from build123d import *

# Parameters (mm, degrees)
SKETCH1_W                     = 32.5
SKETCH1_H                     = 12.4
BOSS_EXTRUDE1_DEPTH           = 5
SKETCH3_W                     = 4.5
SKETCH3_H                     = 12.4
BOSS_EXTRUDE2_DEPTH           = 15.8
SKETCH4_R                     = 1
CUT_EXTRUDE1_DEPTH            = 5
SKETCH5_R                     = 1
BOSS_EXTRUDE3_DEPTH           = 2
BOSS_EXTRUDE3_DRAFT           = 5
BOSS_EXTRUDE3_PROFILE_2_DEPTH = 2
BOSS_EXTRUDE3_PROFILE_2_DRAFT = 5
BOSS_EXTRUDE3_PROFILE_3_DEPTH = 2
BOSS_EXTRUDE3_PROFILE_3_DRAFT = 5
SKETCH6_R                     = 4
BOSS_EXTRUDE4_DEPTH           = 1
SKETCH7_R                     = 1.5
BOSS_EXTRUDE5_DEPTH           = 5
FILLET1_R                     = 1
FILLET2_R                     = 1
FILLET3_R                     = 0.5
SKETCH10_W                    = 1.5
SKETCH10_H                    = 3
CUT_EXTRUDE4_DEPTH            = 34.527041325


with BuildPart() as part:
    # Sketch1 → Boss-Extrude1 (new body)
    with BuildSketch(Plane(origin=(0, 0, 0), x_dir=(1, 0, 0), z_dir=(0, 1, 0))):
        Rectangle(SKETCH1_W, SKETCH1_H)
    extrude(amount=BOSS_EXTRUDE1_DEPTH)

    # Sketch3 → Boss-Extrude2 (add)
    with BuildSketch(Plane(origin=(0, 5, 0), x_dir=(1, 0, 0), z_dir=(0, 1, 0))):
        with Locations((-14, 0)):
            Rectangle(SKETCH3_W, SKETCH3_H)
        with Locations((14, 0)):
            Rectangle(SKETCH3_W, SKETCH3_H)
    extrude(amount=BOSS_EXTRUDE2_DEPTH)

    # Sketch4 → Cut-Extrude1 (cut)
    with BuildSketch(Plane(origin=(0, 20.8, 0), x_dir=(1, 0, 0), z_dir=(0, 1, 0))):
        with Locations(Location((14.1, -0.06, 0), (0, 0, 270))):
            Circle(SKETCH4_R)
        with Locations(Location((-14.1, -0.06, 0), (0, 0, 270))):
            Circle(SKETCH4_R)
    extrude(amount=-CUT_EXTRUDE1_DEPTH, mode=Mode.SUBTRACT)


with BuildPart() as boss_extrude3_tool:
    # Sketch5 → Boss-Extrude3 (with draft: the straight prism first)
    with BuildSketch(Plane(origin=(16.25, 0, 0), x_dir=(0, 0, -1), z_dir=(1, 0, 0))):
        with Locations((0, 17.8)):
            Circle(SKETCH5_R)
    extrude(amount=BOSS_EXTRUDE3_DEPTH)
    # Boss-Extrude3: the draft: its side faces are tilted about the plane it starts from
    boss_extrude3_sides = [boss_extrude3_tool.faces().sort_by_distance(p)[0] for p in [
        (17.25, 17.8, 1),
    ]]
    draft(boss_extrude3_sides, Plane(origin=(16.25, 0, 0), x_dir=(0, 0, -1), z_dir=(1, 0, 0)), BOSS_EXTRUDE3_DRAFT)


with BuildPart() as part_1:
    add(part.part)

    # Boss-Extrude3: add boss_extrude3_tool
    add(boss_extrude3_tool.part)


with BuildPart() as boss_extrude3_profile_2_tool:
    # Sketch5 → Boss-Extrude3 profile 2 (with draft: the straight prism first)
    with BuildSketch(Plane(origin=(16.25, 0, 0), x_dir=(0, 0, -1), z_dir=(1, 0, 0))):
        with Locations((3.2, 12.8)):
            Circle(SKETCH5_R)
    extrude(amount=BOSS_EXTRUDE3_PROFILE_2_DEPTH)
    # Boss-Extrude3 profile 2: the draft: its side faces are tilted about the plane it starts from
    boss_extrude3_profile_2_sides = [boss_extrude3_profile_2_tool.faces().sort_by_distance(p)[0] for p in [
        (17.25, 12.8, -2.2),
    ]]
    draft(boss_extrude3_profile_2_sides, Plane(origin=(16.25, 0, 0), x_dir=(0, 0, -1), z_dir=(1, 0, 0)), BOSS_EXTRUDE3_PROFILE_2_DRAFT)


with BuildPart() as part_2:
    add(part_1.part)

    # Boss-Extrude3 profile 2: add boss_extrude3_profile_2_tool
    add(boss_extrude3_profile_2_tool.part)


with BuildPart() as boss_extrude3_profile_3_tool:
    # Sketch5 → Boss-Extrude3 profile 3 (with draft: the straight prism first)
    with BuildSketch(Plane(origin=(16.25, 0, 0), x_dir=(0, 0, -1), z_dir=(1, 0, 0))):
        with Locations((-3.2, 12.8)):
            Circle(SKETCH5_R)
    extrude(amount=BOSS_EXTRUDE3_PROFILE_3_DEPTH)
    # Boss-Extrude3 profile 3: the draft: its side faces are tilted about the plane it starts from
    boss_extrude3_profile_3_sides = [boss_extrude3_profile_3_tool.faces().sort_by_distance(p)[0] for p in [
        (17.25, 12.8, 4.2),
    ]]
    draft(boss_extrude3_profile_3_sides, Plane(origin=(16.25, 0, 0), x_dir=(0, 0, -1), z_dir=(1, 0, 0)), BOSS_EXTRUDE3_PROFILE_3_DRAFT)


with BuildPart() as part_3:
    add(part_2.part)

    # Boss-Extrude3 profile 3: add boss_extrude3_profile_3_tool
    add(boss_extrude3_profile_3_tool.part)

    # Sketch6 → Boss-Extrude4 (add)
    with BuildSketch(Plane.ZY.offset(16.25)):
        with Locations(Location((0, 17.8, 0), (0, 0, 131.409622109))):
            Circle(SKETCH6_R)
    extrude(amount=BOSS_EXTRUDE4_DEPTH)

    # Sketch7 → Boss-Extrude5 (add)
    with BuildSketch(Plane.ZY.offset(17.25)):
        with Locations((0, 17.8)):
            Circle(SKETCH7_R)
    extrude(amount=BOSS_EXTRUDE5_DEPTH)

    # Fillet1
    fillet1_edges = [part_3.edges().sort_by_distance(p)[0] for p in [
        (-22.25, 17.8, -1.5),
    ]]
    fillet(fillet1_edges, radius=FILLET1_R)

    # Fillet2
    fillet2_edges = [part_3.edges().sort_by_distance(p)[0] for p in [
        (-17.25, 14.8, 2.645751311),
    ]]
    fillet(fillet2_edges, radius=FILLET2_R - 0.0001)  # a hair under: the kernel refuses the full size

    # Fillet3
    fillet3_edges = [part_3.edges().sort_by_distance(p)[0] for p in [
        (18.25, 17.8, 0.825022673),
        (18.25, 12.8, -2.374977327),
        (18.25, 12.8, 4.025022673),
    ]]
    fillet(fillet3_edges, radius=FILLET3_R)

    # Sketch10 → Cut-Extrude4 (cut, through all)
    with BuildSketch(Plane(origin=(0, 0, -6.2), x_dir=(-1, 0, 0), z_dir=(0, 0, -1))):
        with Locations((-12.5, 9)):
            Rectangle(SKETCH10_W, SKETCH10_H)
    extrude(amount=-CUT_EXTRUDE4_DEPTH, mode=Mode.SUBTRACT)


solid = part_3.part
Read the model definition and answer for the solid it produces. Units are mm, in the model's axes. A direction names the side the tool comes from. Round coordinates to 2 decimals unless told otherwise and drop trailing zeros. Write each loop counter-clockwise with the first axis right and the second up, starting at its lowest first coordinate (ties: lowest second). Pieces come first, ordered by that corner, then holes.
1. The part is cut by section A-A, the plane z = 5.25. Determine the outline of the cut face in (x, y), then the cut area to 3 significant figures.
2. Determine the mould class of faces 5 (the face through (13.25, 9, 0)), 6 (the face through (-19.222, 16.336, -0.325)), 7 (the face through (14, 15.8, 0)) for opening direction Z: pulls with the +Z half, pulls with the -Z half, needs draft (parallel to the pull), parting line crosses it, or undercut.
3. Straight lines are drawn through the part: L1, parallel to X at y = 9, z = 0; L2, parallel to Y at x = 12, z = -1.5; L3, parallel to X at y = 12.5, z = 1.25. For each, find the intervals that lie inside material, in ascending order.
4. Given pin 1 Ø1.6 at (x, z) = (14.5, -0.5) entering from +Y; pin 2 Ø6 at (y, z) = (7.5, 0) entering from -X; pin 3 Ø6 at (x, z) = (0.5, 2) entering from +Y, each flat-ended and moving along its own axis, determine where each tip first touches the part or whether it passes through.
5. The part is cut by section C-C, the plane y = 1.5. Determine the outline of the cut face in (x, z).
6. Which of the six approach directions +Z, -Z, +X, -X, +Y, -Y give full straight-line access (tool end or side, diameter ignored) to faces 1 (the face through (13, 7.5, 0)), 2 (the face through (11.75, 16, 0)), 3 (the face through (-13.11, 18.34, -0.07)), 4 (the face through (-16.25, 21, 0))?
7. The part is cut by section B-B, the plane x = 14.1. Determine the outline of the cut face in (y, z), then the cut area to 3 significant figures.
8. The part is cut by section D-D, the plane x = 10. Determine the outline of the cut face in (y, z), then the cut area to 3 significant figures.
Values:
1. outline: (-16.25, 0) - (16.25, 0) - (16.25, 20.8) - (11.75, 20.8) - (11.75, 10.5) - (13.25, 10.5) - (13.25, 7.5) - (11.75, 7.5) - (11.75, 5) - (-11.75, 5) - (-11.75, 20.8) - (-16.25, 20.8) - close
1. area: 300 mm2
2. face 5: needs draft
2. face 6: parting line crosses it
2. face 7: undercut
3. L1: x = -16.25 to -11.75, 13.25 to 16.25
3. L2: y = 0 to 7.5, 10.5 to 20.8
3. L3: x = -16.25 to -11.75, 11.75 to 16.25
4. pin 1: stops at y = 20.8
4. pin 2: stops at x = -16.25
4. pin 3: stops at y = 5
5. outline: (-16.25, -6.2) - (16.25, -6.2) - (16.25, 6.2) - (-16.25, 6.2) - close
6. face 1: +Z, -Z
6. face 2: +Z, -Z, +Y
6. face 3: +Y
6. face 4: +Z, -Z, +X, +Y
7. outline: (0, -6.2) - (20.8, -6.2) - (20.8, -0.94) - (15.8, -0.94) - (15.8, 1.06) - (20.8, 1.06) - (20.8, 6.2) - (0, 6.2) - close
7. area: 248 mm2
8. outline: (0, -6.2) - (5, -6.2) - (5, 6.2) - (0, 6.2) - close
8. area: 62.0 mm2
